from build123d import *

# Parameters (mm, degrees)
SKETCH_1_R                    = 50
EXTRUDE_1_DEPTH               = 3.302
SKETCH_2_R                    = 4.064
CUT_EXTRUDE_1_DEPTH           = 71.787733429
SKETCH_4_R                    = 5.08
CUT_EXTRUDE_3_DEPTH           = 71.787733429
SKETCH_7_R                    = 1.27
CUT_EXTRUDE_6_DEPTH           = 71.787733429
M3_CLEARANCE_HOLE1_AT_2_COUNT = 2
M3_CLEARANCE_HOLE1_AT_2_PITCH = 12.419742348
F_3_8_CLEARANCE_HOLE1_D       = 10.0838
SKETCH11_R                    = 1.5
CUT_EXTRUDE5_DEPTH            = 71.787733429
CIRPATTERN1_COUNT             = 2
CIRPATTERN2_COUNT             = 2
SKETCH12_W                    = 38.1
SKETCH12_H                    = 9.525
CUT_EXTRUDE6_DEPTH            = 71.787733429
FILLET1_R                     = 3.175
FILLET1_OF_MIRROR1_R          = 3.175


with BuildPart() as part:
    # 草图1 → 凸台-拉伸1 (new body)
    with BuildSketch(Plane.XY):
        with Locations(Location((0, 0, 0), (0, 0, 180))):
            Circle(SKETCH_1_R)
    extrude(amount=EXTRUDE_1_DEPTH)

    # 草图2 → 切除-拉伸1 (cut, through all)
    with BuildSketch(Plane.XY.offset(3.302)):
        with Locations((-26.940768363, 26.940768363)):
            Circle(SKETCH_2_R)
        with Locations((-26.940768363, -26.940768363)):
            Circle(SKETCH_2_R)
        with Locations((26.940768363, -26.940768363)):
            Circle(SKETCH_2_R)
        with Locations((26.940768363, 26.940768363)):
            Circle(SKETCH_2_R)
    extrude(amount=-CUT_EXTRUDE_1_DEPTH, mode=Mode.SUBTRACT)

    # 草图4 → 切除-拉伸3 (cut, through all)
    with BuildSketch(Plane.XY.offset(3.302)):
        Circle(SKETCH_4_R)
    extrude(amount=-CUT_EXTRUDE_3_DEPTH, mode=Mode.SUBTRACT)

    # 草图7 → 切除-拉伸6 (cut, through all)
    with BuildSketch(Plane.XY.offset(3.302)):
        with Locations((0, 46.99)):
            Circle(SKETCH_7_R)
        with Locations((46.99, 0)):
            Circle(SKETCH_7_R)
        with Locations((0, -46.99)):
            Circle(SKETCH_7_R)
        with Locations((-46.99, 0)):
            Circle(SKETCH_7_R)
    extrude(amount=-CUT_EXTRUDE_6_DEPTH, mode=Mode.SUBTRACT)

    # Sketch2 → M3 Clearance Hole1 (revolve, cut)
    with BuildSketch(Plane(origin=(0, 8, 3.302), x_dir=(0, -1, 0), z_dir=(1, 0, 0))):
        Polygon((0, 0), (0, 26.421463052), (1.7, 25.4), (1.7, 0), align=None)
    m3_clearance_hole1 = revolve(axis=Axis((0, 8, 9.652), (0, 0, -1)), mode=Mode.SUBTRACT)

    # M3 Clearance Hole1 at 2: M3 Clearance Hole1 ×2
    with Locations(*[Vector(-0.7649111981170567, -0.6441357457827728, 0) * (i * M3_CLEARANCE_HOLE1_AT_2_PITCH) for i in range(1, M3_CLEARANCE_HOLE1_AT_2_COUNT)]):
        add(m3_clearance_hole1, mode=Mode.SUBTRACT)

    # 3/8 Clearance Hole1 (through all)
    with Locations(Plane.XY.offset(3.302)):
        with Locations((0, 31.75), (-31.75, 0), (31.75, 0), (0, -31.75)):
            Hole(F_3_8_CLEARANCE_HOLE1_D / 2)

    # Sketch11 → Cut-Extrude5 (cut, through all)
    with BuildSketch(Plane.XY.offset(3.302)):
        with Locations((-16.51, 0)):
            Circle(SKETCH11_R)
    cut_extrude5 = extrude(amount=-CUT_EXTRUDE5_DEPTH, mode=Mode.SUBTRACT)

    # CirPattern1: Cut-Extrude5 ×2 about axis
    cirpattern1_axis = Axis((0, 0, 0), (0, 0, 1))
    for i in range(1, CIRPATTERN1_COUNT):
        add(cut_extrude5.rotate(cirpattern1_axis, i * 360 / CIRPATTERN1_COUNT), mode=Mode.SUBTRACT)

    # CirPattern2: M3 Clearance Hole1 ×2 about axis
    cirpattern2_axis = Axis((0, 0, 0), (0, 0, 1))
    for i in range(1, CIRPATTERN2_COUNT):
        add(m3_clearance_hole1.rotate(cirpattern2_axis, i * 360 / CIRPATTERN2_COUNT), mode=Mode.SUBTRACT)

    # CirPattern2 copy 1 sketch → CirPattern2 copy 1 (revolve, cut)
    with BuildSketch(Plane(origin=(9.5, 0, 3.302), x_dir=(0, 1, 0), z_dir=(-1, 0, 0))):
        Polygon((0, 0), (0, 26.421463052), (1.7, 25.4), (1.7, 0), align=None)
    revolve(axis=Axis((9.5, 0, 9.652), (0, 0, -1)), mode=Mode.SUBTRACT)

    # Sketch12 → Cut-Extrude6 (cut, through all)
    with BuildSketch(Plane.XY.offset(3.302)):
        with Locations((0, 17.145)):
            Rectangle(SKETCH12_W, SKETCH12_H)
    cut_extrude6 = extrude(amount=-CUT_EXTRUDE6_DEPTH, mode=Mode.SUBTRACT)

    # Fillet1
    fillet1_edges = [part.edges().sort_by_distance(p)[0] for p in [
        (19.05, 21.9075, 1.651),
        (19.05, 12.3825, 1.651),
        (-19.05, 12.3825, 1.651),
        (-19.05, 21.9075, 1.651),
    ]]
    fillet(fillet1_edges, radius=FILLET1_R)

    # Mirror1: Cut-Extrude6 across plane
    add(cut_extrude6.mirror(Plane.ZX), mode=Mode.SUBTRACT)

    # Fillet1 of Mirror1
    fillet1_of_mirror1_edges = [part.edges().sort_by_distance(p)[0] for p in [
        (19.05, -21.9075, 1.651),
        (19.05, -12.3825, 1.651),
        (-19.05, -12.3825, 1.651),
        (-19.05, -21.9075, 1.651),
    ]]
    fillet(fillet1_of_mirror1_edges, radius=FILLET1_OF_MIRROR1_R)


solid = part.part
Part model, mm, in its own coordinate system. Round coordinates to 2 decimals unless told otherwise and drop trailing zeros. Write each loop counter-clockwise with the first axis right and the second up, starting at its lowest first coordinate (ties: lowest second). Pieces come first, ordered by that corner, then holes. Notation, with made-up numbers: M 3,-26.75 L 27,-26.75 A26 cw 27,3.25 Z; hole C -22,43.5 d8. An arc over 180 degrees is marked long. Return JSON: item names as keys, results as strings. Group by question number.
(1) Saw through at C-C on x = 9.5. Write the cut outline in (y, z).
(2) Two-plate mould, pull along X, no slides. Class faces 1 (the face through (19.05, 17, 2)), 2 (the face through (1, 10, 3.302)): +X half, -X half, draft (parallel to the pull), parting line (faces both ways), or undercut.
(3) Saw through at A-A on y = 46.99. Write the cut outline in (x, z), then the cut area to 3 significant figures.
(4) Drill centre lines: probe 1 along Y at (x, z) = (-3, 2.4); probe 2 along Y at (x, z) = (-26.5, 0.85); probe 3 along X at (y, z) = (-17.5, 2.5). Where is each one in solid material? Low to high.
(5) Saw through at D-D on y = 0. Count the separate pieces of the cut face and the enclosed holes in it, then the cut area to 3 significant figures.
(6) Pin check, flat tips, straight feed: pin 1 Ø1.5 at (x, z) = (-5.5, 2) entering from -Y; pin 2 Ø1.6 at (y, z) = (-18, 1) entering from +X. Stop position of each tip, or through.
Returned:
{
 "1": {"outline": "M -49.09,0 L -21.91,0 L -21.91,3.3 L -49.09,3.3 Z; M -12.38,0 L -1.7,0 L -1.7,3.3 L -12.38,3.3 Z; M 1.7,0 L 12.38,0 L 12.38,3.3 L 1.7,3.3 Z; M 21.91,0 L 49.09,0 L 49.09,3.3 L 21.91,3.3 Z"},
 "2": {"face 1": "undercut", "face 2": "draft"},
 "3": {"outline": "M -17.09,0 L -1.27,0 L -1.27,3.3 L -17.09,3.3 Z; M 1.27,0 L 17.09,0 L 17.09,3.3 L 1.27,3.3 Z", "area": "104 mm²"},
 "4": {"probe 1": "-49.91 to -35.8, -27.7 to -21.91, -12.38 to -4.1, 4.1 to 12.38, 21.91 to 27.7, 35.8 to 49.91", "probe 2": "-42.4 to -30.98, -22.9 to 22.9, 30.98 to 42.4", "probe 3": "-46.84 to -19.05, 19.05 to 46.84"},
 "5": {"separate pieces": "10", "enclosed holes": "0", "area": "171 mm²"},
 "6": {"pin 1": "y = -49.77", "pin 2": "x = 46.95"}
}
